from build123d import *

# Parameters (mm, degrees)
SKETCH1_R                   = 7.9375
BOSS_EXTRUDE1_DEPTH         = 57.15
CHAMFER1_SIZE               = 0.254
F_5_16_0_3125_DOWEL_HOLE1_D = 9.525


with BuildPart() as part:
    # Sketch1 → Boss-Extrude1 (new body)
    with BuildSketch(Plane.XY):
        Circle(SKETCH1_R)
    extrude(amount=BOSS_EXTRUDE1_DEPTH)

    # Chamfer1
    chamfer1_edges = [part.edges().sort_by_distance(p)[0] for p in [
        (-7.9375, 0, 57.15),
    ]]
    chamfer(chamfer1_edges, length=CHAMFER1_SIZE)

    # 5/16 (0.3125) Dowel Hole1 (through all)
    with Locations(Plane.XY.offset(57.15)):
        with Locations((0, 0)):
            Hole(F_5_16_0_3125_DOWEL_HOLE1_D / 2)


solid = part.part
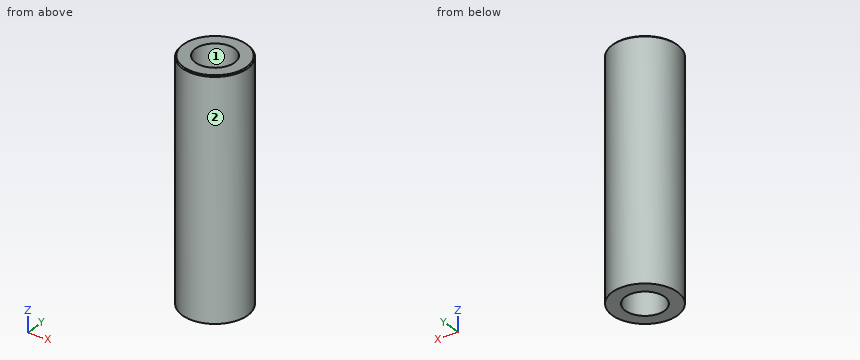
Can you work these out from the model? Positions are in its coordinate system, mm. Face numbers are marked on the shaded views. Round coordinates to 2 decimals unless told otherwise and drop trailing zeros. Write each loop counter-clockwise with the first axis right and the second up, starting at its lowest first coordinate (ties: lowest second). Pieces come first, ordered by that corner, then holes. Notation, with made-up numbers: (73.5, 52) -> (125.5, 52) arc R21 cw to (125.5, 67) -> close; hole circle Ø2 at (70, -16). An arc over 180 degrees is marked (long way). One line per question, with ' | ' between items. Start each with the question number.
1) I need wall thicknesses on line 1 (Y direction, x = -0.25, z = 48); line 2 (X direction, y = 1.5, z = 27); line 3 (X direction, y = 1, z = 8.5). Which ranges of each line are inside material? Lowest first, please. Write a range as [from, to].
2) I'm going to push flat-ended pins straight in: P1, Ø2, axis at y = 4, z = 35, coming from the +X side; P2, Ø1, axis at y = 4.5, z = 33.5, coming from the -X side; P3, Ø6, axis at x = -3.5, z = 26.5, coming from the +Y side. Where does each tip first touch, or does it pass through?
3) Suppose I cut it at A-A on x = 0. Write out the boundary of the cut face in (y, z).
4) Suppose I cut it at B-B on z = 38. Write out the boundary of the cut face in (x, y) (1 decimal).
5) If we mould it in two halves opening along X, with no side actions, what happens to the marked faces 1 and 2? For each: released by +X, released by -X, zero draft, split by the parting line, or undercut.
Return value:
1) line 1: y = [-7.93, -4.76], [4.76, 7.93] | line 2: x = [-7.79, -4.52], [4.52, 7.79] | line 3: x = [-7.87, -4.66], [4.66, 7.87]
2) P1: stops at x = 7.35 | P2: stops at x = -6.86 | P3: stops at y = 7.92
3) outline: (-7.94, 0) -> (-4.76, 0) -> (-4.76, 57.15) -> (-7.68, 57.15) -> (-7.94, 56.9) -> close; (4.76, 0) -> (7.94, 0) -> (7.94, 56.9) -> (7.68, 57.15) -> (4.76, 57.15) -> close
4) outline: circle Ø15.9 at (0, 0); hole circle Ø9.5 at (0, 0)
5) face 1: undercut | face 2: split by the parting line
